```python
from build123d import *

# Parameters (mm, degrees)
F1_DEPTH = 15
F3_DEPTH = 50
F5_DEPTH = 160
F6_R     = 2.5
F7_DEPTH = 15


with BuildPart() as f1:
    # F0 (on Top) → F1 (new body)
    with BuildSketch(Plane.XY):
        Polygon((-15, 0), (15, 0), (15, 25.566243), (80, 63.094011), (80, 140), (60, 140), (60, 74.641016), (0, 40), (-60, 74.641016), (-60, 140), (-80, 140), (-80, 63.094011), (-15, 25.566243), align=None)
    extrude(amount=F1_DEPTH)

    # F2 (on face) → F3 (cut)
    with BuildSketch(Plane.XZ):
        with BuildLine():
            Line((4, 15), (-4, 15))
            ThreePointArc((-4, 15), (0, 11), (4, 15))
        make_face()
    extrude(amount=-F3_DEPTH, mode=Mode.SUBTRACT)

    # F4 (on face) → F5 (cut, through all)
    with BuildSketch(Plane(origin=(-80, 0, 0), x_dir=(0, -1, 0), z_dir=(-1, 0, 0))):
        with BuildLine():
            Line((-125, 15), (-135, 15))
            ThreePointArc((-135, 15), (-130, 10), (-125, 15))
        make_face()
    extrude(amount=-F5_DEPTH, mode=Mode.SUBTRACT)

    # F6 (on face) → F7 (cut, through all)
    with BuildSketch(Plane.XY.offset(15)):
        with Locations((-9.5, 6)):
            Circle(F6_R)
        with Locations((-9.5, 26)):
            Circle(F6_R)
        with Locations((9.5, 6)):
            Circle(F6_R)
        with Locations((9.5, 26)):
            Circle(F6_R)
    extrude(amount=-F7_DEPTH, mode=Mode.SUBTRACT)


solid = f1.part
```
Check sheet for the modelled part. Datum: model origin and axes. Units: mm. A direction names the side the tool comes from. Give positions to 0.01 mm unless a question says otherwise; leave off trailing zeros. Write each loop counter-clockwise with the first axis right and the second up, starting at its lowest first coordinate (ties: lowest second). Pieces come first, ordered by that corner, then holes. Notation, with made-up numbers: (67, 32) - (81, 32) arc R18 cw to (81, 58) - close; hole circle Ø7 at (26, 73). An arc over 180 degrees is marked (long way). Answer as a JSON object with one key per item and string values. Group by question number.
1) Access from +Z, -Z, +X, -X, +Y, -Y to the whole of each face (thin tool, end or side, straight path). Record for faces 1 (the face through (-60, 107, 7)), 2 (the face through (80, 101, 7)), 3 (the face through (-15, 13, 7)).
2) Sectioned sample at D-D (x = -10). Record the cut outline in (y, z).
3) Sectioned sample at C-C (z = 2.5). Record the cut outline in (x, y).
4) Sectioned sample at B-B (y = 6). Record the cut outline in (x, z).
5) Depth check by flat-ended pin: P1, Ø1, axis at x = 44.5, z = 9, coming from the +Y side; P2, Ø8, axis at x = 14, z = 10.5, coming from the +Y side; P3, Ø4.5, axis at y = 18.5, z = 4, coming from the +X side. Enter the tip coordinate at first touch or a pass-through.
6) Release check for a two-part mould opening along Y. For faces 4 (the face through (30.42, 57.563, 7.395)), 5 (the face through (70, 130, 10)), 6 (the face through (-47.95, 44.59, 7.4)), 7 (the face through (-48, 63, 15)) record: pulls with the +Y half, pulls with the -Y half, needs draft (parallel to the pull), parting line crosses it, or undercut.
7) Thickness scan on probe 1 along X at (y, z) = (128, 2.25); probe 2 along Y at (x, z) = (-8.5, 2.5); probe 3 along Y at (x, z) = (9.5, 11.75). Record the ranges inside material, lowest first. Write a range as from..to.
8) Sectioned sample at A-A (y = 130). Record the cut outline in (x, z).
Geometry results:
{
 "1": {"face 1": "+Z, -Z, +Y", "face 2": "+Z, -Z, +X, +Y, -Y", "face 3": "+Z, -Z, -X, -Y"},
 "2": {"outline": "(0, 0) - (3.55, 0) - (3.55, 15) - (0, 15) - close; (8.45, 0) - (23.55, 0) - (23.55, 15) - (8.45, 15) - close; (28.45, 0) - (45.77, 0) - (45.77, 15) - (28.45, 15) - close"},
 "3": {"outline": "(-80, 63.09) - (-15, 25.57) - (-15, 0) - (15, 0) - (15, 25.57) - (80, 63.09) - (80, 140) - (60, 140) - (60, 74.64) - (0, 40) - (-60, 74.64) - (-60, 140) - (-80, 140) - close; hole circle Ø5 at (-9.5, 6); hole circle Ø5 at (-9.5, 26); hole circle Ø5 at (9.5, 6); hole circle Ø5 at (9.5, 26)"},
 "4": {"outline": "(-15, 0) - (-12, 0) - (-12, 15) - (-15, 15) - close; (-7, 0) - (7, 0) - (7, 15) - (4, 15) arc R4 cw to (-4, 15) - (-7, 15) - close; (12, 0) - (15, 0) - (15, 15) - (12, 15) - close"},
 "5": {"P1": "stops at y = 65.98", "P2": "stops at y = 50.39", "P3": "stops at x = 15"},
 "6": {"face 4": "pulls with the +Y half", "face 5": "undercut", "face 6": "pulls with the -Y half", "face 7": "needs draft"},
 "7": {"probe 1": "x = -80..-60, 60..80", "probe 2": "y = 0..3.71, 8.29..23.71, 28.29..44.91", "probe 3": "y = 0..3.5, 8.5..23.5, 28.5..45.48"},
 "8": {"outline": "(-80, 0) - (-60, 0) - (-60, 10) - (-80, 10) - close; (60, 0) - (80, 0) - (80, 10) - (60, 10) - close"}
}
